```python
from build123d import *

# Parameters (mm, degrees)
SKETCH1_R                    = 14.5
BOSS_EXTRUDE1_DEPTH          = 4
SKETCH2_R                    = 15
BOSS_EXTRUDE2_DEPTH          = 8
SKETCH3_R                    = 13
BOSS_EXTRUDE3_DEPTH          = 16
SKETCH4_R                    = 15
BOSS_EXTRUDE4_DEPTH          = 4.5
SKETCH5_R                    = 12.5
BOSS_EXTRUDE5_DEPTH          = 0.5
SKETCH6_R                    = 13
BOSS_EXTRUDE6_DEPTH          = 5.25
SKETCH7_R                    = 11
CUT_EXTRUDE1_DEPTH           = 5.5
SKETCH8_R                    = 10
CUT_EXTRUDE2_DEPTH           = 32.75
FILLET1_R                    = 0.75
CHAMFER1_SIZE                = 0.5
F_2_0_2_DIAMETER_HOLE3_D     = 2
F_2_0_2_DIAMETER_HOLE3_DEPTH = 8.649139381
F_2_0_2_DIAMETER_HOLE3_TIP   = 0.600860619


with BuildPart() as part:
    # Sketch1 → Boss-Extrude1 (new body)
    with BuildSketch(Plane.XY):
        Circle(SKETCH1_R)
    extrude(amount=BOSS_EXTRUDE1_DEPTH)

    # Sketch2 → Boss-Extrude2 (add)
    with BuildSketch(Plane.XY.offset(4)):
        Circle(SKETCH2_R)
    extrude(amount=BOSS_EXTRUDE2_DEPTH)

    # Sketch3 → Boss-Extrude3 (add)
    with BuildSketch(Plane.XY.offset(12)):
        Circle(SKETCH3_R)
    extrude(amount=BOSS_EXTRUDE3_DEPTH)

    # Sketch4 → Boss-Extrude4 (add)
    with BuildSketch(Plane.XY.offset(28)):
        Circle(SKETCH4_R)
    extrude(amount=BOSS_EXTRUDE4_DEPTH)

    # Sketch5 → Boss-Extrude5 (add)
    with BuildSketch(Plane.XY.offset(32.5)):
        Circle(SKETCH5_R)
    extrude(amount=BOSS_EXTRUDE5_DEPTH)

    # Sketch6 → Boss-Extrude6 (add)
    with BuildSketch(Plane.XY.offset(33)):
        Circle(SKETCH6_R)
    extrude(amount=BOSS_EXTRUDE6_DEPTH)

    # Sketch7 → Cut-Extrude1 (cut)
    with BuildSketch(Plane.XY.offset(38.25)):
        Circle(SKETCH7_R)
    extrude(amount=-CUT_EXTRUDE1_DEPTH, mode=Mode.SUBTRACT)

    # Sketch8 → Cut-Extrude2 (cut)
    with BuildSketch(Plane.XY.offset(32.75)):
        with Locations((-1.44, 0.75)):
            Circle(SKETCH8_R)
    extrude(amount=-CUT_EXTRUDE2_DEPTH, mode=Mode.SUBTRACT)

    # Fillet1
    fillet1_edges = [part.edges().sort_by_distance(p)[0] for p in [
        (-13, 0, 12),
        (-13, 0, 28),
    ]]
    fillet(fillet1_edges, radius=FILLET1_R)

    # Chamfer1
    chamfer1_edges = [part.edges().sort_by_distance(p)[0] for p in [
        (-13, 0, 38.25),
    ]]
    chamfer(chamfer1_edges, length=CHAMFER1_SIZE)

    # Ø2.0 (2) Diameter Hole3
    with Locations(Plane(origin=(0, 0, 0), x_dir=(-1, 0, 0), z_dir=(0, 0, -1))):
        with Locations((-9.5, 8.8)):
            Hole(F_2_0_2_DIAMETER_HOLE3_D / 2, depth=F_2_0_2_DIAMETER_HOLE3_DEPTH)
            with Locations((0, 0, -(F_2_0_2_DIAMETER_HOLE3_DEPTH + F_2_0_2_DIAMETER_HOLE3_TIP / 2))):  # 118° drill point
                Cone(0, F_2_0_2_DIAMETER_HOLE3_D / 2, F_2_0_2_DIAMETER_HOLE3_TIP, mode=Mode.SUBTRACT)


solid = part.part
```
Geometry: final body of the model. Coordinates: model frame, mm. A direction names the side the tool comes from. Coordinates: 2 decimals unless noted, no trailing zeros. Loops run counter-clockwise (first coordinate to the right, second up) from the corner with the lowest first, then second, coordinate; pieces in that order, holes last. Notation, with made-up numbers: M 30,-7.5 L 59,-7.5 A11 ccw 59,7.5 Z; hole C 26,-9.5 d10. An arc over 180 degrees is marked long. Put each result on its own line as item: value.
(1) Draft query along X for faces 4 (the face through (-10.316, -7.91, 19.898)), 5 (the face through (-2.38, -10.74, 35.54)), 6 (the face through (-3.4, 12.3, 32.5)). Return one class per face: pulls with the +X half, pulls with the -X half, needs draft (parallel to the pull), parting line crosses it, or undercut.
Answer sheet:
face 4: parting line crosses it
face 5: undercut
face 6: needs draft
(2) First-contact query: pin 1 (4 mm diameter, centred on x = -3, z = 34, fed in from +Y); pin 2 (3 mm diameter, centred on x = 8, z = 23, fed in from +Y); pin 3 (1 mm diameter, centred on x = 10, z = 24, fed in from -Y). Flat tips, straight axial feed; report the tip coordinate or a pass-through.
Answer sheet:
pin 1: stops at y = 14.91
pin 2: stops at y = 11.26
pin 3: stops at y = -8.87
(3) Material intervals for probe 1 along Z at (x, y) = (9.5, -11); probe 2 along X at (y, z) = (-3.5, 18); probe 3 along Y at (x, z) = (-9.5, 26), sorted ascending.
Answer sheet:
probe 1: z = 4 to 12, 28 to 32.5
probe 2: x = -12.52 to -10.49, 7.61 to 12.52
probe 3: y = -8.87 to -5.17, 6.67 to 8.87
(4) Cut plane A-A on z = 2. Return the cut outline in (x, y).
Answer sheet:
outline: C 0,0 d29; hole C -1.44,0.75 d20; hole C 9.5,8.8 d2
(5) Access query for faces 1 (the face through (8.7, 8.2, 4.4)), 2 (the face through (-10.316, -7.91, 35.342)), 3 (the face through (-6.8, 10.7, 33)). Directions: +Z, -Z, +X, -X, +Y, -Y. A direction counts if a zero-diameter tool reaches every point of the face in a straight line with its end or side. Return the directions, or none.
Answer sheet:
face 1: -Z
face 2: +Z
face 3: none
